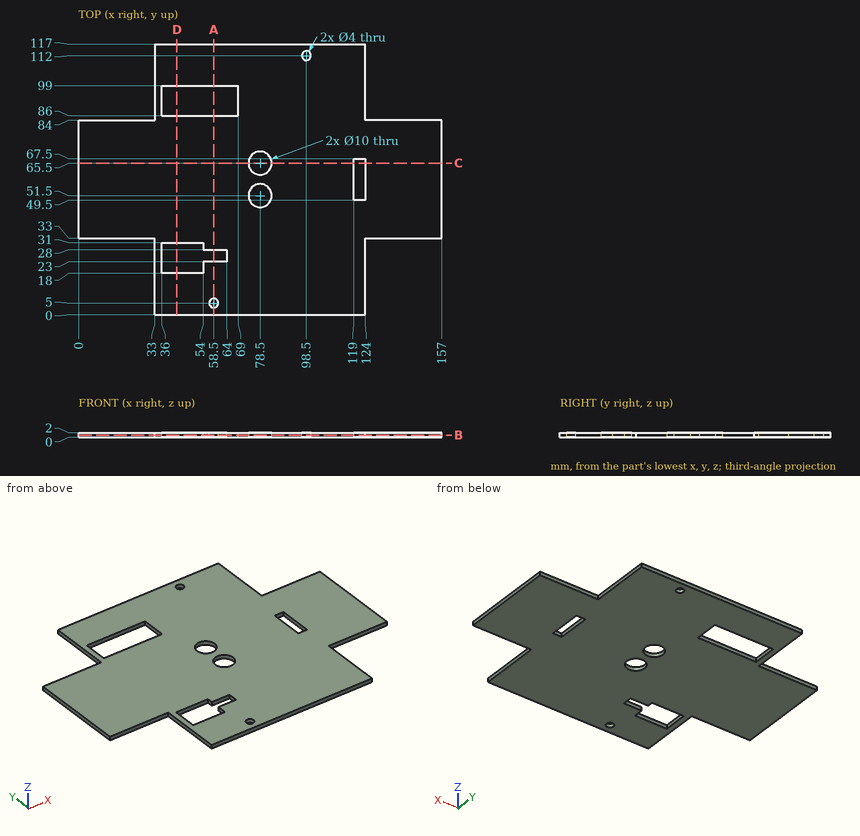
Here's the drawing with two shaded views (mm, measured from the low corner). I have some questions. Give positions to 0.01 mm unless a question says otherwise; leave off trailing zeros. Write each loop counter-clockwise with the first axis right and the second up, starting at its lowest first coordinate (ties: lowest second). Pieces come first, ordered by that corner, then holes. Notation, with made-up numbers: (76, 1) -> (125, 1) arc R25 cw to (125, 29) -> close; hole circle Ø3 at (-33, -28.75). An arc over 180 degrees is marked (long way). Use one line per item in the form item = value. Start each with the question number.
1. Imagine slicing it at A-A on x = 58.5. List the corners of the cut face in (y, z) for me, plus the area to 3 significant figures.
2. Imagine slicing it at C-C on y = 65.5. List the corners of the cut face in (x, z) for me.
3. Imagine slicing it at B-B on z = 0.95. State how many separate pieces and enclosed holes the cut face has, plus the area to 3 significant figures.
4. Will these pins go through, and if not, where does the flat tip stop? pin 1 Ø0.6 at (y, z) = (21, 0.5) entering from -X; pin 2 Ø0.6 at (x, z) = (14, 0.5) entering from -Y; pin 3 Ø0.6 at (x, z) = (21.5, 0.5) entering from +Y.
5. Imagine slicing it at D-D on x = 42.5. List the corners of the cut face in (y, z) for me, plus the area to 3 significant figures.
6. If I drill on L1, parallel to Y at x = 78.5, z = 1.3; L2, parallel to Y at x = 58.5, z = 1.2; L3, parallel to X at y = 65.5, z = 1.2, over which ranges is the centre line in solid material (lowest first)?
Entries:
q1.outline = (0, 0) -> (3, 0) -> (3, 2) -> (0, 2) -> close; (7, 0) -> (23, 0) -> (23, 2) -> (7, 2) -> close; (28, 0) -> (86, 0) -> (86, 2) -> (28, 2) -> close; (99, 0) -> (117, 0) -> (117, 2) -> (99, 2) -> close
q1.area = 190 mm²
q2.outline = (0, 0) -> (73.5, 0) -> (73.5, 2) -> (0, 2) -> close; (83.5, 0) -> (119, 0) -> (119, 2) -> (83.5, 2) -> close; (124, 0) -> (157, 0) -> (157, 2) -> (124, 2) -> close
q3.separate_pieces = 1
q3.enclosed_holes = 7
q3.area = 13,000 mm²
q4.pin_1 = 33
q4.pin_2 = 33
q4.pin_3 = 84
q5.outline = (0, 0) -> (18, 0) -> (18, 2) -> (0, 2) -> close; (31, 0) -> (86, 0) -> (86, 2) -> (31, 2) -> close; (99, 0) -> (117, 0) -> (117, 2) -> (99, 2) -> close
q5.area = 182 mm²
q6.L1 = 0 to 46.5, 56.5 to 60.5, 70.5 to 117
q6.L2 = 0 to 3, 7 to 23, 28 to 86, 99 to 117
q6.L3 = 0 to 73.5, 83.5 to 119, 124 to 157
